Input: part model. Units: mm. Frame: model coordinates. Face numbers are marked on the shaded views. A direction names the side the tool comes from. Give positions to 0.01 mm unless a question says otherwise; leave off trailing zeros. Loops run counter-clockwise (first coordinate to the right, second up) from the corner with the lowest first, then second, coordinate; pieces in that order, holes last. Notation, with made-up numbers: (-14, 78) - (37, 78) arc R18 cw to (37, 103) - close; hole circle Ø7 at (75, 12). An arc over 180 degrees is marked (long way). Answer as a JSON object with one key per item and string values.
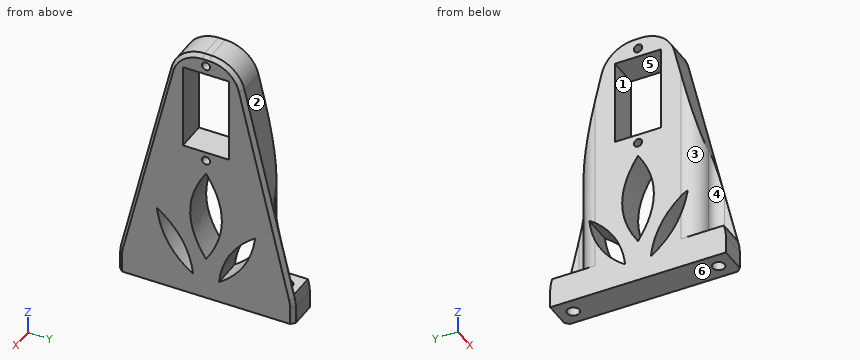
from build123d import *

# Parameters (mm, degrees)
SKETCH1_W           = 8.000974829
SKETCH1_H           = 46.5
BOSS_EXTRUDE1_DEPTH = 70
CUT_EXTRUDE1_DEPTH  = 70
SKETCH3_R           = 1.1
CUT_EXTRUDE2_DEPTH  = 70
FILLET1_R           = 9
CUT_EXTRUDE3_DEPTH  = 62
SKETCH5_R           = 1.6
CUT_EXTRUDE4_DEPTH  = 62
FILLET2_R           = 5
CHAMFER1_SIZE       = 1


with BuildPart() as part:
    # Sketch1 → Boss-Extrude1 (new body)
    with BuildSketch(Plane.XY):
        with Locations((34.458782271, 0)):
            Rectangle(SKETCH1_W, SKETCH1_H)
    extrude(amount=BOSS_EXTRUDE1_DEPTH)

    # Sketch2 → Cut-Extrude1 (cut)
    with BuildSketch(Plane(origin=(38.459269685, 0, 0), x_dir=(0, 0, -1), z_dir=(1, 0, 0))):
        with BuildLine():
            Line((0, -23.25), (-4.675968949, -23.25))
            ThreePointArc((-4.675968949, -23.25), (-5.84025075, -23.181991134), (-6.988696254, -22.978889578))
            Line((-6.988696254, -22.978889578), (-70, -8))
            Line((-70, -8), (-70, 0))
            Line((-70, 0), (-70, 8))
            Line((-70, 8), (-6.988696254, 22.978889578))
            ThreePointArc((-6.988696254, 22.978889578), (-5.84025075, 23.181991134), (-4.675968949, 23.25))
            Line((-4.675968949, 23.25), (0, 23.25))
            Line((0, 23.25), (0, 33.462731107))
            Line((0, 33.462731107), (-74.824697051, 33.462731107))
            Line((-74.824697051, 33.462731107), (-74.824697051, -41.354226456))
            Line((-74.824697051, -41.354226456), (0, -41.354226456))
            Line((0, -41.354226456), (0, -23.25))
        make_face()
        with BuildLine():
            add(Edge.make_bspline(
                [(-36.048150351, 0), (-23.713645553, -8.388071288), (-11.218940507, 0)],
                knots=[0, 0, 0, 1, 1, 1], degree=2))
            add(Edge.make_bspline(
                [(-36.048150351, 0), (-23.713645553, 8.388071288), (-11.218940507, 0)],
                knots=[0, 0, 0, 1, 1, 1], degree=2))
        make_face()
        with BuildLine():
            add(Edge.make_bspline(
                [(-5.680368735, 3.40627966), (-15.724909711, 4.511710031), (-21.714178832, 13.021085274)],
                knots=[0, 0, 0, 1, 1, 1], degree=2))
            add(Edge.make_bspline(
                [(-5.680368735, 3.40627966), (-11.386784663, 11.746039667), (-21.714178832, 13.021085274)],
                knots=[0, 0, 0, 1, 1, 1], degree=2))
        make_face()
        with BuildLine():
            add(Edge.make_bspline(
                [(-5.680368735, -3.40627966), (-15.724909711, -4.511710031), (-21.714178832, -13.021085274)],
                knots=[0, 0, 0, 1, 1, 1], degree=2))
            add(Edge.make_bspline(
                [(-5.680368735, -3.40627966), (-11.386784663, -11.746039667), (-21.714178832, -13.021085274)],
                knots=[0, 0, 0, 1, 1, 1], degree=2))
        make_face()
    extrude(amount=-CUT_EXTRUDE1_DEPTH, mode=Mode.SUBTRACT)

    # Sketch3 → Cut-Extrude2 (cut)
    with BuildSketch(Plane.ZY.offset(-30.458294856)):
        with Locations((67.2, 0)):
            Circle(SKETCH3_R)
        with Locations(Location((39.8, 0, 0), (0, 0, 270))):
            Circle(SKETCH3_R)
        Polygon((53.5, 6.1), (42.15, 6.1), (42.15, -6.1), (64.85, -6.1), (64.85, 6.1), align=None)
    extrude(amount=-CUT_EXTRUDE2_DEPTH, mode=Mode.SUBTRACT)

    # Fillet1
    fillet1_edges = [part.edges().sort_by_distance(p)[0] for p in [
        (34.458782271, -8, 70),
        (34.458782271, 8, 70),
    ]]
    fillet(fillet1_edges, radius=FILLET1_R)

    # Sketch4 → Cut-Extrude3 (cut)
    with BuildSketch(Plane.XY.offset(70)):
        with BuildLine():
            ThreePointArc((37.397007822, -19.25), (36.536421482, -17.172360788), (34.458782271, -16.311774449))
            Line((34.458782271, -16.311774449), (30.458294856, -16.311774449))
            Line((30.458294856, -16.311774449), (30.458294856, -22.188225551))
            Line((30.458294856, -22.188225551), (30.458294856, -24.738187672))
            Line((30.458294856, -24.738187672), (37.397007822, -23.25))
            Line((37.397007822, -23.25), (37.397007822, -19.25))
        make_face()
        with BuildLine():
            Line((30.458294856, 24.500594278), (30.458294856, 22.188225551))
            Line((30.458294856, 22.188225551), (30.458294856, 16.311774449))
            Line((30.458294856, 16.311774449), (34.458782271, 16.311774449))
            ThreePointArc((34.458782271, 16.311774449), (36.536421482, 17.172360788), (37.397007822, 19.25))
            Line((37.397007822, 19.25), (37.397007822, 23.25))
            Line((37.397007822, 23.25), (30.458294856, 24.500594278))
        make_face()
    extrude(amount=-CUT_EXTRUDE3_DEPTH, mode=Mode.SUBTRACT)

    # Sketch5 → Cut-Extrude4 (cut)
    with BuildSketch(Plane.XY.offset(8)):
        with Locations((34.458782271, 19.25)):
            Circle(SKETCH5_R)
        with Locations((34.458782271, -19.25)):
            Circle(SKETCH5_R)
    extrude(amount=-CUT_EXTRUDE4_DEPTH, mode=Mode.SUBTRACT)

    # Fillet2
    # the kernel refuses this fillet: 5 mm, written as the material it takes off along each edge
    with BuildSketch(Plane(origin=(30.458294856, -16.311774449, 56.016575811), x_dir=(0, 1, 0), z_dir=(0, 0, -1))) as fillet2_piece_1:
        with BuildLine():
            CenterArc((4.936823623, 5), FILLET2_R, 187.233387323, 82.766612677)
            Line((-0.023383871, 4.37044332), (-0.519404621, 4.307487652))
            ThreePointArc((-0.519404621, 4.307487652), (-0.5, 4.000487415), (-0.5, 0))
            Line((-0.5, 0), (0, -0.5))
            Line((0, -0.5), (4.936823623, -0.5))
            Line((4.936823623, -0.5), (4.936823623, 0))
        make_face()
    extrude(amount=48.016575811, mode=Mode.SUBTRACT)
    with BuildSketch(Plane(origin=(30.458294856, 16.311774449, 56.016575811), x_dir=(0, -1, 0), z_dir=(0, 0, -1))) as fillet2_piece_2:
        with BuildLine():
            CenterArc((4.936823623, -5), FILLET2_R, 90, 82.766612677)
            Line((-0.023383871, -4.37044332), (-0.519404621, -4.307487652))
            ThreePointArc((-0.519404621, -4.307487652), (-0.5, -4.000487415), (-0.5, 0))
            Line((-0.5, 0), (0, 0.5))
            Line((0, 0.5), (4.936823623, 0.5))
            Line((4.936823623, 0.5), (4.936823623, 0))
        make_face()
    extrude(amount=48.016575811, mode=Mode.SUBTRACT)

    # Chamfer1
    chamfer1_edges = [part.edges().sort_by_distance(p)[0] for p in [
        (38.459269685, 16.311774449, 35.035075414),
        (38.459269685, 0, 70),
        (38.459269685, -6.468394753, 68.061624854),
        (38.459269685, 6.468394753, 68.061624854),
        (38.459269685, 23.25, 2.337984474),
        (38.459269685, -23.25, 2.337984474),
        (38.459269685, -23.181991134, 5.84025075),
        (38.459269685, -16.311774449, 35.035075414),
        (38.459269685, 23.181991134, 5.84025075),
    ]]
    chamfer(chamfer1_edges, length=CHAMFER1_SIZE)


solid = part.part
Item 1: Access query for the marked faces 1, 2 and 3. Directions: +Z, -Z, +X, -X, +Y, -Y. A direction counts if a zero-diameter tool reaches every point of the face in a straight line with its end or side. Return the directions, or none.
Geometry check:
{"face 1": "+X, -X", "face 2": "+Z, +X, -X, +Y", "face 3": "+Z, -X, -Y"}
Item 2: Mould query, pull axis Y, two halves, no side actions, for the marked faces 4, 5 and 6. Classes: released by +Y, released by -Y, zero draft, split by the parting line, or undercut.
Geometry check:
{"face 4": "released by -Y", "face 5": "undercut", "face 6": "zero draft"}
Item 3: Cut plane B-B (y = 5). Give the number of separate pieces and of enclosed holes in the cut face, then the cut area to 3 significant figures.
Geometry check:
{"separate pieces": "3", "enclosed holes": "0", "area": "329 mm2"}
Item 4: Cut plane A-A (z = 39.8). Return loops of the section in (x, y).
Geometry check:
{"outline": "(30.46, -11.37) arc R5 ccw to (32.21, -15.18) - (37.46, -15.18) - (38.46, -14.15) - (38.46, -1.1) - (30.46, -1.1) - close; (30.46, 1.1) - (38.46, 1.1) - (38.46, 14.15) - (37.46, 15.18) - (32.21, 15.18) arc R5 ccw to (30.46, 11.37) - close"}
Item 5: Contact query for flat-ended pins moving along their axis: P1, Ø2, axis at x = 36, z = 49.5, coming from the -Y side; P2, Ø2.5, axis at x = 34.5, z = 54, coming from the -Y side; P3, Ø1, axis at x = 34.5, z = 32, coming from the -Y side. Output: stop coordinate, or through.
Geometry check:
{"P1": "stops at y = -13.11", "P2": "stops at y = -12.1", "P3": "stops at y = -16.36"}
Item 6: Material intervals for line 1 (Y direction, x = 34.75, z = 21); line 2 (Y direction, x = 35.5, z = 10); line 3 (X direction, y = 19, z = 6), sorted ascending. Write a range as [from, to].
Geometry check:
{"line 1": "y = [-16.32, -12.92], [-12.05, -4], [4, 12.05], [12.92, 16.32]", "line 2": "y = [-16.5, -8.18], [-4.28, 4.28], [8.18, 16.5]", "line 3": "x = [30.46, 32.88], [36.04, 38.46]"}
Item 7: Cut plane C-C (z = 59.5). Return loops of the section in (x, y).
Geometry check:
{"outline": "(30.46, -10.5) - (37.46, -10.5) - (38.46, -9.47) - (38.46, -6.1) - (30.46, -6.1) - close; (30.46, 6.1) - (38.46, 6.1) - (38.46, 9.47) - (37.46, 10.5) - (30.46, 10.5) - close"}
